Can you work these out from the model? Positions are in its coordinate system, mm. Face numbers are marked on the shaded views. A direction names the side the tool comes from. Give positions to 0.01 mm unless a question says otherwise; leave off trailing zeros. Order: outer loops, then holes, each group sorted by start corner. A loop starts at its lowest first (then second) coordinate and runs counter-clockwise, first axis right, second up. Notation, with made-up numbers: (81, 25) - (85, 25) arc R27 cw to (85, 44) - close; hole circle Ø2 at (18.5, 5.25). An arc over 180 degrees is marked (long way). Answer as CSV lines item,"result".
Autodesk Inventor part; units mm, degrees
ref_plane "Work Plane1" through (104.775, 0, 0) normal (0, 0, -1) x (1, 0, 0)
ref_plane "YZ Plane" through (0, 0, 0) normal (1, 0, 0) x (0, 1, 0)
ref_plane "XZ Plane" through (0, 0, 0) normal (0, 1, 0) x (-1, 0, 0)
sketch "Sketch1" plane through (0, 0, 0) normal (0, 0, 1) x (1, 0, 0)
  line L0 (10, 0) -> (10, 1.5)
  line L1 (10, 1.5) -> (3.36, 1.5)
  line L2 (3.36, 1.5) -> (3.0533, 1.5)
  line L3 (0, 2.77) -> (0, 1.1547)
  line L4 (0, 1.1547) -> (1.1, 1.1547)
  line L5 (1.1, 1.1547) -> (1.7667, 0)
  line L6 (1.7667, 0) -> (10, 0)
  line L7 (0, 2.77) -> (0.59, 2.77)
  line L8 (0.59, 2.77) -> (1.86, 1.5)
  line L9 (3.0533, 1.5) -> (1.86, 1.5)
  line L10 (3.36, 1.5) -> (1.86, 1.5) construction
  line L11 (1.86, 1.5) -> (1.86, 1.5)
  line L12 (-2, 0) -> (12, 0)
  line L13 (0, -0.554) -> (0, 3.324)
  dimension "d0" = 10
  dimension "d1" = 6.64
  dimension "d2" = 1.1
  dimension "d3" = 3
  dimension "d6" = 1.86
  dimension "d7" = 45
  dimension "d8" = 2.3094
  dimension "d9" = 60
  dimension "d10" = 5.54
  dimension "d11" = 3
  dimension "d12" = 0.3067
revolve "Body" add sketch "Sketch1" angle 360 about axis through (1.7667, 0, 0) along (1, 0, 0) contours L6 L5 L4 L3 L7 L8 L9 L2 L1 L0
sketch "Sketch2" plane through (0, 0, 0) normal (-1, 0, 0) x (0, 0, 1)
  circle A0 centre (0, 0) radius 1.1547
  line L0 (0, -3.878) -> (0, 3.878)
  line L1 (-3.878, 0) -> (3.878, 0)
  line L2 (1.1547, 0) -> (0.5774, -1)
  line L3 (0.5774, -1) -> (-0.5774, -1)
  line L4 (-0.5774, -1) -> (-1.1547, 0)
  line L5 (-1.1547, 0) -> (-0.5774, 1)
  line L6 (-0.5774, 1) -> (0.5774, 1)
  line L7 (0.5774, 1) -> (1.1547, 0)
  point P0 (0, 1.1547)
extrude "Slot" add sketch "Sketch2" against normal up to next contours L7 A0 | A0 L2 | L6 L0 A0 | A0 L0 L3 | L0 L6 A0 | A0 L3 L0 | L4 A0 | A0 L5
thread "Thread"
chamfer "Chamfer1" distance 0.3067 distance2 0.3067 1 edges at (10, -1.5, 0) measured on face at (10, -0.8298, -0.2045)
ref_plane "Work Plane1" through (104.775, 0, 0) normal (0, 0, -1) x (1, 0, 0)
equation "\"d15\" = GEL"
equation "\"d17\" = -0.5 * SPD + 0.5 * GD"
equation "\"d18\" = GUL"
equation "\"d0\" = NLG"
equation "\"d1\" = GEL"
equation "\"d2\" = INTI"
equation "\"d3\" = GD"
equation "\"d6\" = KOH"
equation "\"d7\" = 0.5 * SEWI"
equation "\"d8\" = 1.1547 * SW"
equation "\"d10\" = KOD"
equation "\"d11\" = BDM"
equation "\"d12\" = GAL"
equation "\"NLG\" = 10"
equation "\"INTI\" = 1.1"
equation "\"GEL\" = 6.64"
equation "\"GAL\" = 0.61345 * PTC"
equation "\"KOH\" = 1.86"
equation "\"KOD\" = 5.54"
equation "\"GUL\" = 0.61345 * PTC"
equation "\"SPD\" = NND - 1.2269 * PTC"
equation "\"BDM\" = NND"
equation "\"GD\" = NND"
equation "\"SEWI\" = 90deg"
equation "\"SW\" = 2"
equation "\"TOA\" = 30deg"
equation "\"GD1\" = THREADDIA - 1.2269 * PTC"
equation "\"EPV\" = 3.36"
equation "\"THREADDIA\" = 3"
equation "\"PTC\" = 0.5"
equation "\"NND\" = 3"
equation "\"E0\" = 2.31"
properties part number "ISO 10642  - M3  x  10" material "Steel"
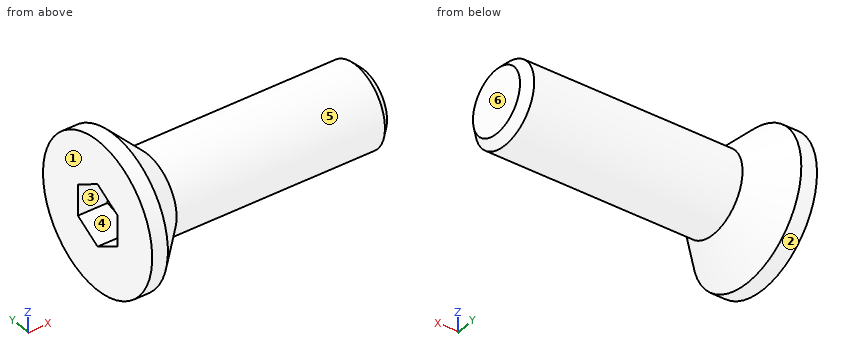
1) Which directions (+Z, -Z, +X, -X, +Y, -Y) give clear straight access to the entire face, cutting with the end or side of a thin tool? Please do the marked faces 4, 5 and 6.
Answer block:
face 4,"-X"
face 5,"+X"
face 6,"+Z, -Z, +X, +Y, -Y"
2) I want a section at A-A on x = 4.5. Write out the boundary of the cut face in (y, z).
Answer block:
outline,"circle Ø3 at (0, 0)"
3) I need wall thicknesses on line 1 along Z through (x, y) = (3.75, -0.1); line 2 along X through (y, z) = (-0.8, 2.3); line 3 along X through (y, z) = (0.85, -1.6). Which ranges of each line are inside material? Lowest first, please. Write a range as [from, to].
Answer block:
line 1,"[-1.5, 1.5]"
line 2,"[0, 0.92]"
line 3,"[0, 1.55]"
4) I'm going to push flat-ended pins straight in: P1, Ø1.5, axis at x = 6.5, z = 2, coming from the +Y side; P2, Ø1.5, axis at y = 1.5, z = -0.5, coming from the -X side. Where does each tip first touch, or does it pass through?
Answer block:
P1,"y = 0.83"
P2,"x = 0"
5) If we mould it in two halves opening along Y, with no side actions, what happens to the marked faces 1, 2 and 3? For each: +Y half, -Y half, draft (parallel to the pull), parting line (faces both ways), or undercut.
Answer block:
face 1,"draft"
face 2,"parting line"
face 3,"undercut"
